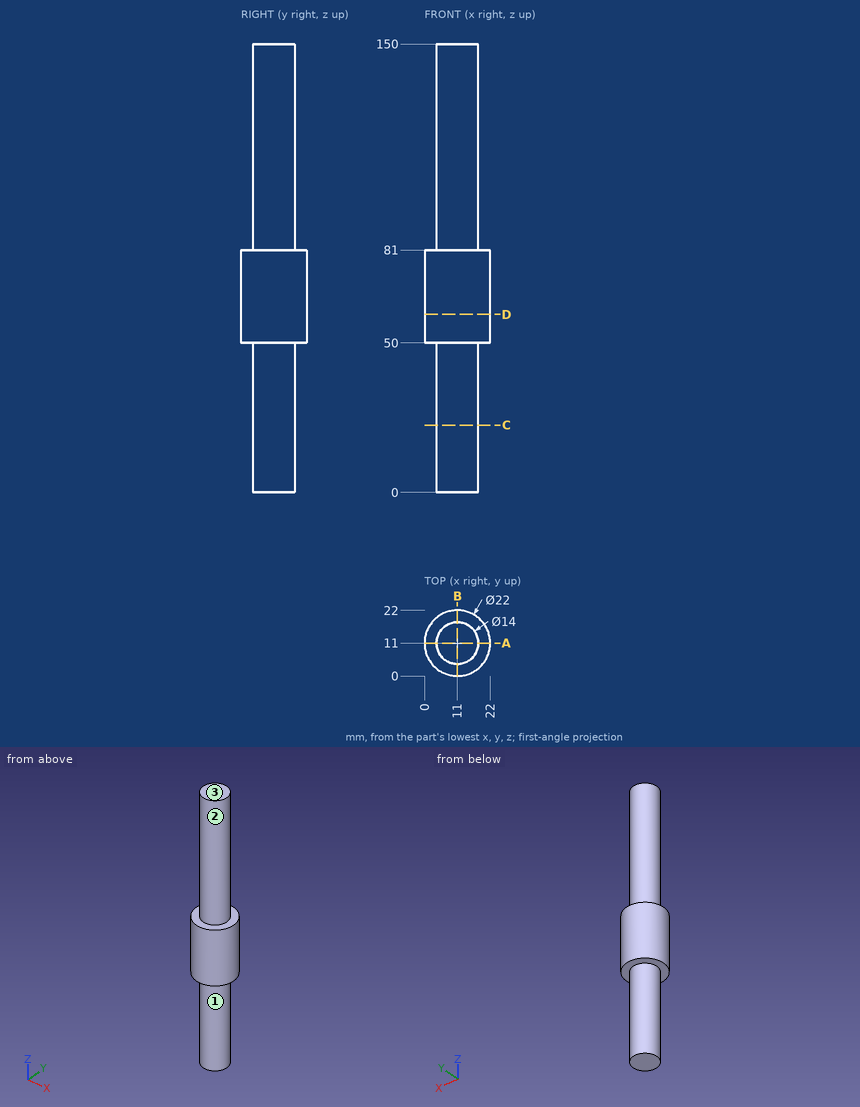
Geometry check sheet. Reference: drawing and pictorial views, mm from the part's lowest x, y, z. A direction names the side the tool comes from. Round coordinates to 2 decimals unless told otherwise and drop trailing zeros. Loops run counter-clockwise (first coordinate to the right, second up) from the corner with the lowest first, then second, coordinate; pieces in that order, holes last. Notation, with made-up numbers: (79.25, 44.5) -> (133.25, 44.5) arc R11 ccw to (133.25, 53.5) -> close; hole circle Ø4 at (72.5, 88.5). An arc over 180 degrees is marked (long way). Use a Markdown table: item, result.
(1) Sectioned sample at C-C (z = 22.5). Enter the section's corners in (x, y).
Calculated:
| item | result |
|---|---|
| outline | circle Ø14 at (11, 11) |
(2) Go/stop test with flat-tipped pins: P1, Ø10, axis at y = 11, z = 131.5, coming from the -X side; P2, Ø5, axis at x = 8, z = 108.5, coming from the -Y side; P3, Ø8, axis at x = 6, z = 94, coming from the +Y side. Record where each tip stops, or that it passes through.
Calculated:
| item | result |
|---|---|
| P1 | x = 4 |
| P2 | y = 4.02 |
| P3 | y = 17.93 |
(3) Sectioned sample at D-D (z = 59.5). Enter the section's corners in (x, y), then the cut area to 3 significant figures.
Calculated:
| item | result |
|---|---|
| outline | circle Ø22 at (11, 11) |
| area | 380 mm² |
(4) Scan lines: probe 1 along Z at (x, y) = (14.75, 2); probe 2 along Y at (x, z) = (16.75, 114); probe 3 along X at (y, z) = (9, 114.5). Record each from-to range of solid material in increasing order.
Calculated:
| item | result |
|---|---|
| probe 1 | 50 to 81 |
| probe 2 | 7.01 to 14.99 |
| probe 3 | 4.29 to 17.71 |
(5) Sectioned sample at A-A (y = 11). Enter the section's corners in (x, z).
Calculated:
| item | result |
|---|---|
| outline | (0, 50) -> (4, 50) -> (4, 0) -> (18, 0) -> (18, 50) -> (22, 50) -> (22, 81) -> (18, 81) -> (18, 150) -> (4, 150) -> (4, 81) -> (0, 81) -> close |
(6) Set-up check for the marked faces 1, 2 and 3: record each of +Z, -Z, +X, -X, +Y, -Y from which the full face is reachable in a straight line by a thin tool's end or side.
Calculated:
| item | result |
|---|---|
| face 1 | -Z |
| face 2 | +Z |
| face 3 | +Z, +X, -X, +Y, -Y |
